CAD build for the part. Positions are in the model's coordinates, mm. Face numbers are marked on the shaded views. A direction names the side the tool comes from. Round coordinates to 2 decimals unless told otherwise and drop trailing zeros. Order: outer loops, then holes, each group sorted by start corner. A loop starts at its lowest first (then second) coordinate and runs counter-clockwise, first axis right, second up. Notation, with made-up numbers: (83, -24) -> (114, -24) arc R14 cw to (114, -17) -> close; hole circle Ø10 at (65.5, -11.5). An arc over 180 degrees is marked (long way). Return JSON: item names as keys, results as strings. Group by question number.
Q1. Cut at C-C (y = -2.75). Count the separate pieces of the cut face and the enclosed holes in it, then the cut area to 3 significant figures.
Q2. Flat gauge pins, fed straight in: pin 1 (1.5 mm diameter, centred on x = 15.5, z = -2, fed in from -Y); pin 2 (8 mm diameter, centred on y = -0.5, z = -12.5, fed in from +X); pin 3 (3 mm diameter, centred on x = 13, y = 2, fed in from -Z). Where does each tip first touch, or does it go through?
Q3. Probe line 1 along X through (y, z) = (-1, -2); line 2 along Z through (x, y) = (18, 1.5); line 3 along X through (y, z) = (-0.5, -2). List the from-to ranges inside material, lowest first.
Q4. Cut at A-A (x = 10.5). Write the cut outline in (y, z) (3 decimals), then the cut area to 3 significant figures.
Q5. Which spindle directions (+Z, -Z, +X, -X, +Y, -Y) get a long thin tool onto all of the face, cutting with end or side? Do the marked faces 1, 2 and 3. Say none if no direction does.
Q6. Cut at B-B (z = -1). Write the cut outline in (x, y) (3 decimals), then the cut area to 3 significant figures.
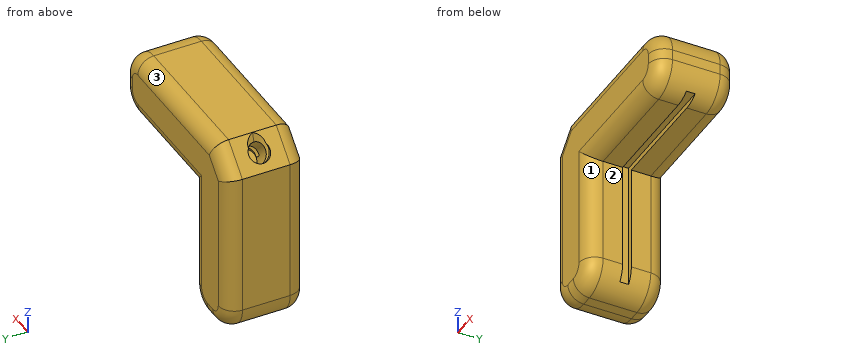
from build123d import *

# Parameters (mm, degrees)
BOSS_EXTRUDE1_DEPTH = 7.5
SKETCH3_W           = 25
SKETCH3_H           = 1.65
CUT_EXTRUDE1_DEPTH  = 1
SKETCH4_W           = 1
SKETCH4_H           = 1.65
CUT_EXTRUDE2_DEPTH  = 26
FILLET1_R           = 5
FILLET2_R           = 3
SKETCH5_R           = 2
CUT_EXTRUDE3_DEPTH  = 7
CUT_SWEEP1_PITCH    = 5


with BuildPart() as part:
    # Sketch1 → Boss-Extrude1 (new, symmetric)
    with BuildSketch(Plane(origin=(0, 0, 0), x_dir=(1, 0, 0), z_dir=(0, 1, 0))):
        Polygon((0, 25), (0, 0), (25, 0), (25, -12), (-7, -12), (-12, -7), (-12, 25), align=None)
    extrude(amount=BOSS_EXTRUDE1_DEPTH, both=True)

    # Sketch3 → Cut-Extrude1 (cut)
    with BuildSketch(Plane(origin=(0, 0, 0), x_dir=(-1, 0, 0), z_dir=(0, 0, -1))):
        with Locations((-12.5, 0)):
            Rectangle(SKETCH3_W, SKETCH3_H)
    extrude(amount=-CUT_EXTRUDE1_DEPTH, mode=Mode.SUBTRACT)

    # Sketch4 → Cut-Extrude2 (cut)
    with BuildSketch(Plane(origin=(0, 0, -25), x_dir=(-1, 0, 0), z_dir=(0, 0, -1))):
        with Locations((0.5, 0)):
            Rectangle(SKETCH4_W, SKETCH4_H)
    extrude(amount=-CUT_EXTRUDE2_DEPTH, mode=Mode.SUBTRACT)

    # Fillet1
    fillet1_edges = [part.edges().sort_by_distance(p)[0] for p in [
        (25, -4.1625, 0),
        (25, 0, 12),
        (0, 4.1625, -25),
        (-12, 0, -25),
    ]]
    fillet(fillet1_edges, radius=FILLET1_R - 0.0001)  # a hair under: the kernel refuses the full size

    # Fillet2
    fillet2_edges = [part.edges().sort_by_distance(p)[0] for p in [
        (-9.5, 7.5, 9.5),
        (6.50005, 7.5, 12),
        (0, 7.5, -10.00005),
        (10.00005, -7.5, 0),
        (-6, -7.5, -25),
        (25, -7.5, 6),
        (-12, -7.5, -6.50005),
        (-10.535563195, -7.5, -23.535563195),
        (-1.464436908, -7.5, -23.535563298),
        (23.535563195, -7.5, 10.535563195),
        (23.535563195, -7.5, 1.464436805),
        (25, 7.5, 6),
        (-6, 7.5, -25),
        (-12, 7.5, -6.50005),
        (10.00005, 7.5, 0),
        (-10.535563195, 7.5, -23.535563195),
        (-1.464436805, 7.5, -23.535563195),
        (23.535563195, 7.5, 10.535563195),
        (23.535563195, 7.5, 1.464436805),
        (0, -7.5, -10.000050146),
        (6.50005, -7.5, 12),
        (-9.5, -7.5, 9.5),
    ]]
    fillet(fillet2_edges, radius=FILLET2_R)

    # Sketch5 → Cut-Extrude3 (cut)
    with BuildSketch(Plane(origin=(-9.5, 0, 9.5), x_dir=(0.7071067811865475, 0, 0.7071067811865477), z_dir=(-0.7071067811865477, 0, 0.7071067811865475))):
        Circle(SKETCH5_R)
    extrude(amount=-CUT_EXTRUDE3_DEPTH, mode=Mode.SUBTRACT)

    # Cut-Sweep1: arcs per turn and ends read off the stored shape
    # Cut-Sweep1: the profile of Sketch8 screwed along a right-hand helix through 2.25 turns, 12 arcs to a turn; built about Z, then put on its axis
    cut_sweep1_z = Axis((0, 0, 0), (0, 0, 1))
    cut_sweep1_corners = [(2, 0, -4.25), (3.5, 0, -5), (2, 0, -5.75), (2, 0, -5)]
    with BuildLine(mode=Mode.PRIVATE) as cut_sweep1_profile:
        Line(cut_sweep1_corners[0], cut_sweep1_corners[1])
        Line(cut_sweep1_corners[1], cut_sweep1_corners[2])
        Line(cut_sweep1_corners[2], cut_sweep1_corners[3])
        Line(cut_sweep1_corners[3], cut_sweep1_corners[0])
    cut_sweep1_cap = Face(cut_sweep1_profile.wire())
    cut_sweep1_turn_angles = [0, 15, 30, 45, 60, 75, 90, 105, 120, 135, 150, 165, 180, 195, 210, 225, 240, 255, 270, 285, 300, 315, 330, 345, 360]
    cut_sweep1_turn_weights = [1, 0.9659258262890683, 1, 0.9659258262890683, 1, 0.9659258262890683, 1, 0.9659258262890683, 1, 0.9659258262890683, 1, 0.9659258262890683, 1, 0.9659258262890683, 1, 0.9659258262890683, 1, 0.9659258262890683, 1, 0.9659258262890683, 1, 0.9659258262890683, 1, 0.9659258262890683, 1]
    cut_sweep1_turn_rails = [Edge.make_bspline([Vector(p[0], p[1], 0).rotate(cut_sweep1_z, cut_sweep1_turn_angles[k]) / cut_sweep1_turn_weights[k] + Vector(0, 0, p[2] + CUT_SWEEP1_PITCH * cut_sweep1_turn_angles[k] / 360) for k in range(25)], [0, 0, 0, 1, 1, 2, 2, 3, 3, 4, 4, 5, 5, 6, 6, 7, 7, 8, 8, 9, 9, 10, 10, 11, 11, 12, 12, 12], 2, cut_sweep1_turn_weights) for p in cut_sweep1_corners]
    cut_sweep1_turn_sides = [Face.make_surface_from_curves(cut_sweep1_turn_rails[p[0]], cut_sweep1_turn_rails[p[1]]) for p in [(0, 1), (1, 2), (2, 3), (3, 0)]]
    cut_sweep1_last_angles = [720, 735, 750, 765, 780, 795, 810]
    cut_sweep1_last_weights = [1, 0.9659258262890683, 1, 0.9659258262890683, 1, 0.9659258262890683, 1]
    cut_sweep1_last_rails = [Edge.make_bspline([Vector(p[0], p[1], 0).rotate(cut_sweep1_z, cut_sweep1_last_angles[k]) / cut_sweep1_last_weights[k] + Vector(0, 0, p[2] + CUT_SWEEP1_PITCH * cut_sweep1_last_angles[k] / 360) for k in range(7)], [0, 0, 0, 1, 1, 2, 2, 3, 3, 3], 2, cut_sweep1_last_weights) for p in cut_sweep1_corners]
    cut_sweep1_last_sides = [Face.make_surface_from_curves(cut_sweep1_last_rails[p[0]], cut_sweep1_last_rails[p[1]]) for p in [(0, 1), (1, 2), (2, 3), (3, 0)]]
    cut_sweep1 = Plane(origin=(-9.5, 0, 9.5), x_dir=(0.7071067811865475, 0, 0.7071067811865477), z_dir=(0.7071067811865477, 0, -0.7071067811865475)) * Solid(Shell([*[p.moved(Location((0, 0, CUT_SWEEP1_PITCH * i))) for i in range(2) for p in cut_sweep1_turn_sides], *cut_sweep1_last_sides, cut_sweep1_cap, cut_sweep1_cap.rotate(cut_sweep1_z, 810).moved(Location((0, 0, CUT_SWEEP1_PITCH * 810 / 360)))]))
    add(cut_sweep1, mode=Mode.SUBTRACT)


solid = part.part
Solution:
{
 "1": {"separate pieces": "1", "enclosed holes": "2", "area": "707 mm²"},
 "2": {"pin 1": "passes through", "pin 2": "stops at x = 0", "pin 3": "stops at z = 0"},
 "3": {"line 1": "x = -12 to 0", "line 2": "z = 0 to 12", "line 3": "x = -12 to -1"},
 "4": {"outline": "(-7.5, 3) arc R3 ccw to (-4.5, 0) -> (-0.825, 0) -> (-0.825, 1) -> (0.825, 1) -> (0.825, 0) -> (4.5, 0) arc R3 ccw to (7.5, 3) -> (7.5, 9) arc R3 ccw to (4.5, 12) -> (-4.5, 12) arc R3 ccw to (-7.5, 9) -> close", "area": "171 mm²"},
 "5": {"face 1": "-Z, +X, -Y", "face 2": "-Z, +X, +Y, -Y", "face 3": "+Z, +X, -X, +Y"},
 "6": {"outline": "(-12, -4.5) arc R3 ccw to (-9, -7.5) -> (-3, -7.5) arc R3 ccw to (0, -4.5) -> (0, -0.825) -> (-1, -0.825) -> (-1, 0.825) -> (0, 0.825) -> (0, 4.5) arc R3 ccw to (-3, 7.5) -> (-9, 7.5) arc R3 ccw to (-12, 4.5) -> close", "area": "171 mm²"}
}
